The listing builds one solid part. Answer for the finished solid, in the listing's coordinates (mm). Give positions to 0.01 mm unless a question says otherwise; leave off trailing zeros. Write each loop counter-clockwise with the first axis right and the second up, starting at its lowest first coordinate (ties: lowest second). Pieces come first, ordered by that corner, then holes. Notation, with made-up numbers: (80, 37) - (139, 37) arc R20 ccw to (139, 48) - close; hole circle Ø1 at (36.5, -33.75). An arc over 180 degrees is marked (long way). One line per question, with ' | ' between items. Start each with the question number.
1. Given P1, Ø0.6, axis at y = 1, z = 0.5, coming from the -X side, flat-ended and moving along its own axis, determine where the tip first touches the part or whether it passes through.
2. A cutting plane is placed at C-C (z = 0.5). State how many separate pieces and enclosed holes the cut face has, then the cut area to 3 significant figures.
3. A cutting plane is placed at A-A (x = 2). Determine the outline of the cut face in (y, z).
4. A cutting plane is placed at B-B (x = 13). Determine the outline of the cut face in (y, z), then the cut area to 3 significant figures.
5. Find the intervals of material crossed by L1, parallel to Y at x = -30, z = 1.55; L2, parallel to Y at x = 30, z = 1.55; L3, parallel to X at y = 0.5, z = 0.5, in increasing order. Write a range as from..to.
```python
from build123d import *

# Parameters (mm, degrees)
SKETCH_1_W              = 75
SKETCH_1_H              = 15
EXTRUDE_1_DEPTH         = 2
FILLET_1_R              = 7.5
SKETCH_2_R              = 2
SKETCH_2_R_2            = 4.5
CUT_EXTRUDE_1_DEPTH     = 2
CUT_EXTRUDE_2_DEPTH     = 10
FILLET_2_R              = 1
CUT_EXTRUDE_START       = -34
CUT_EXTRUDE_3_OUTLINE_W = 11
CUT_EXTRUDE_3_OUTLINE_H = 4
CUT_EXTRUDE_3_DEPTH     = 2.625249005
FILLET_3_R              = 1


with BuildPart() as part:
    # 草图1 → 凸台-拉伸1 (new body)
    with BuildSketch(Plane.XY):
        Rectangle(SKETCH_1_W, SKETCH_1_H)
    extrude(amount=EXTRUDE_1_DEPTH)

    # 圆角1
    fillet_1_edges = [part.edges().sort_by_distance(p)[0] for p in [
        (37.5, -7.5, 1),
        (-37.5, -7.5, 1),
        (-37.5, 7.5, 1),
        (37.5, 7.5, 1),
    ]]
    fillet(fillet_1_edges, radius=FILLET_1_R - 0.0001)  # a hair under: the kernel refuses the full size

    # 草图2 → 切除-拉伸1 (cut)
    with BuildSketch(Plane.XY.offset(2)):
        with Locations((30, 0)):
            Circle(SKETCH_2_R)
        with Locations((-30, 0)):
            Circle(SKETCH_2_R_2)
    extrude(amount=-CUT_EXTRUDE_1_DEPTH, mode=Mode.SUBTRACT)

    # 草图3 → 切除-拉伸2 (cut)
    with BuildSketch(Plane.XY.offset(2)):
        Polygon((-20, -3.969223594), (-20, 3.969223594), (-4.123105626, 0), align=None)
        Polygon((-15.876894374, 5), (0, 1.030776406), (15.876894374, 5), align=None)
        Polygon((0, -1.030776406), (-15.876894374, -5), (15.876894374, -5), align=None)
        Polygon((4.123105626, 0), (20, -3.969223594), (20, 3.969223594), align=None)
    extrude(amount=-CUT_EXTRUDE_2_DEPTH, mode=Mode.SUBTRACT)

    # 圆角2
    fillet_2_edges = [part.edges().sort_by_distance(p)[0] for p in [
        (-20, -3.969223594, 1),
        (-20, 3.969223594, 1),
        (-4.123105626, 0, 1),
        (0, -1.030776406, 1),
        (15.876894374, -5, 1),
        (-15.876894374, -5, 1),
        (4.123105626, 0, 1),
        (20, 3.969223594, 1),
        (20, -3.969223594, 1),
        (0, 1.030776406, 1),
        (-15.876894374, 5, 1),
        (15.876894374, 5, 1),
    ]]
    fillet(fillet_2_edges, radius=FILLET_2_R)

    # 切除-拉伸3: read off the stored shape, not the designer's step
    # 切除-拉伸3 outline → 切除-拉伸3 (cut)
    with BuildSketch(Plane(origin=(0, 0, 0), x_dir=(0.5477225575051656, 0.8366600265340758, 0), z_dir=(0.8366600265340758, -0.5477225575051659, 0)).offset(CUT_EXTRUDE_START)):
        with Locations((-16.5, 1)):
            Rectangle(CUT_EXTRUDE_3_OUTLINE_W, CUT_EXTRUDE_3_OUTLINE_H)
    extrude(amount=CUT_EXTRUDE_3_DEPTH, mode=Mode.SUBTRACT)

    # 圆角3
    fillet_3_edges = [part.edges().sort_by_distance(p)[0] for p in [
        (-32.999968349, 6.87391189, 1),
        (-37.5, 0, 1),
    ]]
    fillet(fillet_3_edges, radius=FILLET_3_R)


solid = part.part
```
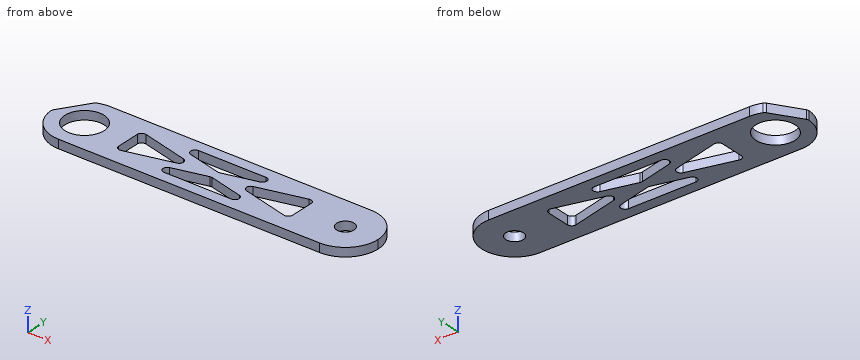
Determined:
1) P1: x = -37.04
2) separate pieces: 1 | enclosed holes: 6 | area: 775 mm2
3) outline: (-7.5, 0) - (-5, 0) - (-5, 2) - (-7.5, 2) - close; (-1.53, 0) - (1.53, 0) - (1.53, 2) - (-1.53, 2) - close; (5, 0) - (7.5, 0) - (7.5, 2) - (5, 2) - close
4) outline: (-7.5, 0) - (-2.22, 0) - (-2.22, 2) - (-7.5, 2) - close; (2.22, 0) - (7.5, 0) - (7.5, 2) - (2.22, 2) - close | area: 21.1 mm2
5) L1: -7.5..-4.5, 4.5..7.5 | L2: -7.5..-2, 2..7.5 | L3: -37.17..-34.47, -25.53..-20, -7.38..7.38, 20..28.06, 31.94..37.48
